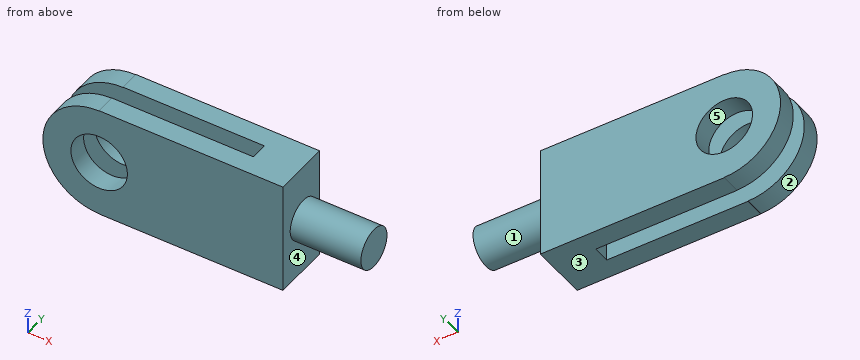
```python
from build123d import *

# Parameters (mm, degrees)
F0_R     = 10
F1_DEPTH = 20
F2_W     = 74.504801
F2_H     = 6
F3_DEPTH = 40
F4_R     = 7.126224
F5_DEPTH = 25


with BuildPart() as f1:
    # F0 (on Front) → F1 (new body)
    with BuildSketch(Plane.XZ):
        with BuildLine():
            Line((-65, 0), (0, 0))
            Line((0, 0), (0, 40))
            Line((0, 40), (-65, 40))
            Line((-65, 40), (-65, 39.89539))
            ThreePointArc((-65, 39.89539), (-84.89539, 20), (-65, 0.10461))
            Line((-65, 0.10461), (-65, 0))
        make_face()
        with Locations((-65, 20)):
            Circle(F0_R, mode=Mode.SUBTRACT)
    extrude(amount=F1_DEPTH)

    # F2 (on face) → F3 (cut, through all)
    with BuildSketch(Plane.XY.offset(40)):
        with Locations((-52.252401, -10)):
            Rectangle(F2_W, F2_H)
    extrude(amount=-F3_DEPTH, mode=Mode.SUBTRACT)

    # F4 (on face) → F5 (join)
    with BuildSketch(Plane.YZ):
        with Locations((-8.923112, 20)):
            Circle(F4_R)
    extrude(amount=F5_DEPTH)


solid = f1.part
```
For this review, take the finished solid that the model builds, in its own axes (mm). Face numbers are marked on the shaded views. A direction names the side the tool comes from. Coordinates: 2 decimals unless noted, no trailing zeros. Write each loop counter-clockwise with the first axis right and the second up, starting at its lowest first coordinate (ties: lowest second). Pieces come first, ordered by that corner, then holes.
(1) Add section C-C on x = -73. Give the boundary of the cut face in (y, z).
(2) Add section D-D on z = 32.5. Give the boundary of the cut face in (x, y), then the cut area to 3 significant figures.
(3) For pin 1 Ø5 at (y, z) = (-11.5, 11.5) entering from -X; pin 2 Ø8 at (y, z) = (-13, 14.5) entering from -X; pin 3 Ø6.5 at (y, z) = (-10.5, 13) entering from -X, all flat-tipped, find the tip position at first contact; note any pin that passes through.
(4) The part is to be moulded in two halves that separate along X. For the marked faces 3, 4 and 5, say which applies: +X half, -X half, draft (parallel to the pull), parting line (faces both ways), or undercut.
(5) Add section A-A on x = -43.5. Give the boundary of the cut face in (y, z).
(6) Wall thickness on probe 1 along X at (y, z) = (-3, 20); probe 2 along Y at (x, z) = (-16, 11.5); probe 3 along Z at (x, y) = (-57.5, -2): over which ranges is each line inside the solid? List them lowest first.
(7) Tool access review of the marked faces 1 and 2: name each direction out of +Z, -Z, +X, -X, +Y, -Y from which nothing blocks a thin tool from reaching the whole face with its end or side.
(8) Add section B-B on z = 20. Give the boundary of the cut face in (x, y), then the cut area to 3 significant figures.
Answer sheet:
1. outline: (-20, 1.78) - (-13, 1.78) - (-13, 14) - (-20, 14) - close; (-20, 26) - (-13, 26) - (-13, 38.22) - (-20, 38.22) - close; (-7, 1.78) - (0, 1.78) - (0, 14) - (-7, 14) - close; (-7, 26) - (0, 26) - (0, 38.22) - (-7, 38.22) - close
2. outline: (-80.48, -20) - (0, -20) - (0, 0) - (-80.48, 0) - (-80.48, -7) - (-15, -7) - (-15, -13) - (-80.48, -13) - close
2. area: 1,220 mm2
3. pin 1: stops at x = -83.8
3. pin 2: stops at x = -84.84
3. pin 3: stops at x = -84.28
4. face 3: draft
4. face 4: +X half
4. face 5: undercut
5. outline: (-20, 0) - (-13, 0) - (-13, 40) - (-20, 40) - close; (-7, 0) - (0, 0) - (0, 40) - (-7, 40) - close
6. probe 1: x = -84.9 to -75, -55 to 25
6. probe 2: y = -20 to -13, -7 to 0
6. probe 3: z = 0 to 13.39, 26.61 to 40
7. face 1: +X
7. face 2: -X, +Y, -Y
8. outline: (-84.9, -20) - (-75, -20) - (-75, -13) - (-84.9, -13) - close; (-84.9, -7) - (-75, -7) - (-75, 0) - (-84.9, 0) - close; (-55, -20) - (0, -20) - (0, -16.05) - (25, -16.05) - (25, -1.8) - (0, -1.8) - (0, 0) - (-55, 0) - (-55, -7) - (-15, -7) - (-15, -13) - (-55, -13) - close
8. area: 1,350 mm2
